CAD build for the part. Positions are in the model's coordinates, mm. Face numbers are marked on the shaded views. Give positions to 0.01 mm unless a question says otherwise; leave off trailing zeros. Write each loop counter-clockwise with the first axis right and the second up, starting at its lowest first coordinate (ties: lowest second). Pieces come first, ordered by that corner, then holes. Notation, with made-up numbers: (71, 18) -> (123, 18) arc R35 cw to (123, 50) -> close; hole circle Ø9 at (-12, 23). An arc over 180 degrees is marked (long way). Answer as a JSON object with one key per item and string values.
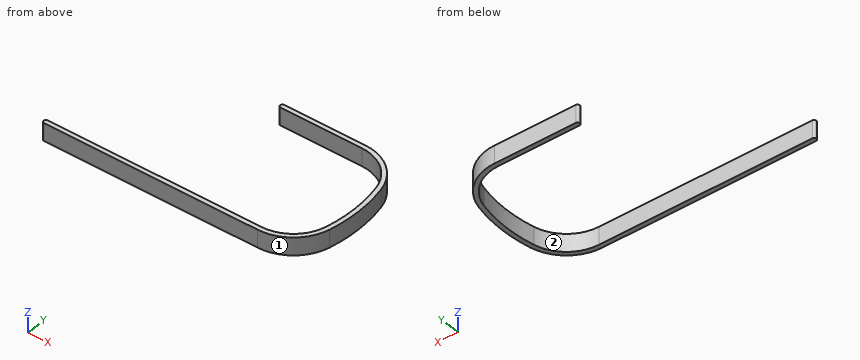
```python
from build123d import *

# Parameters (mm, degrees)
BOSS_EXTRUDE1_DEPTH = 40


with BuildPart() as part:
    # Sketch1 → Boss-Extrude1 (new body)
    with BuildSketch(Plane.XY):
        with BuildLine():
            Line((-5.802272282, 50), (174.679242578, 50))
            ThreePointArc((174.679242578, 50), (237.215894164, 28.0331161), (272.277838453, -28.216655834))
            ThreePointArc((272.277838453, -28.216655834), (280.191261544, -100), (272.277838453, -171.783344166))
            ThreePointArc((272.277838453, -171.783344166), (237.215894164, -228.0331161), (174.679242578, -250))
            Line((174.679242578, -250), (-300, -250))
            ThreePointArc((-300, -250), (-305, -245), (-300, -240))
            Line((-300, -240), (174.679242578, -240))
            ThreePointArc((174.679242578, -240), (230.962229006, -220.22980449), (262.517978866, -169.60500975))
            ThreePointArc((262.517978866, -169.60500975), (270.191261544, -100), (262.517978866, -30.39499025))
            ThreePointArc((262.517978866, -30.39499025), (230.962229006, 20.22980449), (174.679242578, 40))
            Line((174.679242578, 40), (-5.802272282, 40))
            ThreePointArc((-5.802272282, 40), (-10.802272282, 45), (-5.802272282, 50))
        make_face()
    extrude(amount=BOSS_EXTRUDE1_DEPTH)


solid = part.part
```
1) Slice it at D-D (x = -118.5). List the corners of the cut face in (y, z), then the cut area to 3 significant figures.
Model answer:
{"outline": "(-250, 0) -> (-240, 0) -> (-240, 40) -> (-250, 40) -> close", "area": "400 mm2"}
2) Slice it at B-B (z = 25.5). List the corners of the cut face in (x, y) (3 decimals).
Model answer:
{"outline": "(-300, -250) -> (174.679, -250) arc R100 ccw to (272.278, -171.783) arc R329.533 ccw to (272.278, -28.217) arc R100 ccw to (174.679, 50) -> (-5.802, 50) arc R5 ccw to (-5.802, 40) -> (174.679, 40) arc R90 cw to (262.518, -30.395) arc R319.533 cw to (262.518, -169.605) arc R90 cw to (174.679, -240) -> (-300, -240) arc R5 ccw to start"}
3) Slice it at A-A (x = 33). List the corners of the cut face in (y, z).
Model answer:
{"outline": "(-250, 0) -> (-240, 0) -> (-240, 40) -> (-250, 40) -> close; (40, 0) -> (50, 0) -> (50, 40) -> (40, 40) -> close"}
4) Wall check: probe 1 along Y at (x, z) = (140, 23); probe 2 along Y at (x, z) = (-92, 37); probe 3 along Y at (x, z) = (215, 2). Give the ranges that are in metal, low to high.
Model answer:
{"probe 1": "y = -250 to -240, 40 to 50", "probe 2": "y = -250 to -240", "probe 3": "y = -241.51 to -230.46, 30.46 to 41.51"}
5) Mould opens along Y. For the marked faces 1 and 2 say: released by +Y, released by -Y, zero draft, split by the parting line, or undercut.
Model answer:
{"face 1": "released by -Y", "face 2": "undercut"}
6) Slice it at C-C (y = -5.5). List the corners of the cut face in (x, z), then the cut area to 3 significant figures.
Model answer:
{"outline": "(252.91, 0) -> (264.23, 0) -> (264.23, 40) -> (252.91, 40) -> close", "area": "453 mm2"}
7) Pin check, flat tips, straight feed: pin 1 (3 mm diameter, centred on y = 17, z = 25, fed in from +X); pin 2 (1.5 mm diameter, centred on y = -194.5, z = 17.5, fed in from -X); pin 3 (5 mm diameter, centred on y = -127.5, z = 17, fed in from +X). Stop position of each tip, or through.
Model answer:
{"pin 1": "stops at x = 250.24", "pin 2": "stops at x = 252.48", "pin 3": "stops at x = 279.24"}
